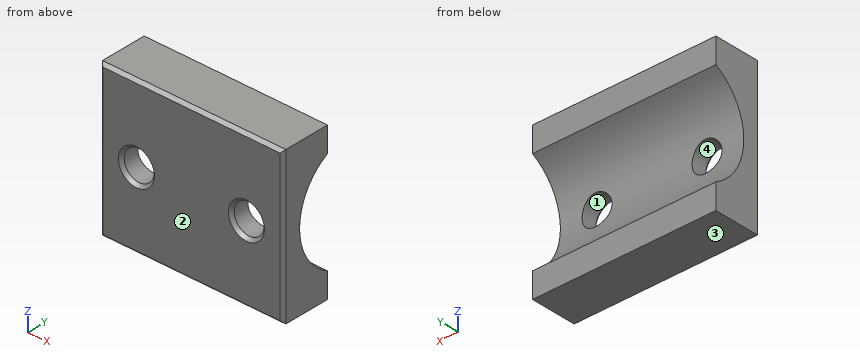
from build123d import *

# Parameters (mm, degrees)
BOSS_EXTRUDE1_DEPTH     = 15
CUT_EXTRUDE1_DEPTH      = 22.100947846
CUT_EXTRUDE1_DEPTH_BACK = 22.100947846
SKETCH2_R               = 2.45
CHAMFER1_SIZE           = 0.5


with BuildPart() as part:
    # Sketch1 → Boss-Extrude1 (new, symmetric)
    with BuildSketch(Plane(origin=(0, 0, 0), x_dir=(0, 0, -1), z_dir=(1, 0, 0))):
        with BuildLine():
            Line((-8.394976176, -4.5), (-12.5, -4.5))
            Line((-12.5, -4.5), (-12.5, -12.5))
            Line((-12.5, -12.5), (12.5, -12.5))
            Line((12.5, -12.5), (12.5, -4.5))
            Line((12.5, -4.5), (8.394976176, -4.5))
            ThreePointArc((8.394976176, -4.5), (0, -9.525), (-8.394976176, -4.5))
        make_face()
    extrude(amount=BOSS_EXTRUDE1_DEPTH, both=True)

    # Sketch2 → Cut-Extrude1 (cut, two sides: drawn at the far end of the back side and taken through both)
    with BuildSketch(Plane.XZ.offset(12.5).offset(-CUT_EXTRUDE1_DEPTH_BACK)):
        with Locations(Location((9, 0, 0), (0, 0, 270))):
            Circle(SKETCH2_R)
        with Locations(Location((-9, 0, 0), (0, 0, 270))):
            Circle(SKETCH2_R)
    extrude(amount=CUT_EXTRUDE1_DEPTH + CUT_EXTRUDE1_DEPTH_BACK, mode=Mode.SUBTRACT)

    # Chamfer1
    chamfer1_edges = [part.edges().sort_by_distance(p)[0] for p in [
        (0, -12.5, -12.5),
        (0, -12.5, 12.5),
        (15, -12.5, 0),
        (-9, -12.5, 2.45),
        (9, -12.5, 2.45),
        (-15, -12.5, 0),
    ]]
    chamfer(chamfer1_edges, length=CHAMFER1_SIZE)


solid = part.part
Part model, mm, in its own coordinate system. Face numbers are marked on the shaded views. Round coordinates to 2 decimals unless told otherwise and drop trailing zeros. Write each loop counter-clockwise with the first axis right and the second up, starting at its lowest first coordinate (ties: lowest second). Pieces come first, ordered by that corner, then holes. Notation, with made-up numbers: M -29,-16.5 L 24,-16.5 A31 ccw 24,11.5 Z; hole C 6.5,40.5 d2. An arc over 180 degrees is marked long. Return JSON: item names as keys, results as strings. Group by question number.
(1) Saw through at D-D on x = 13.5. Write the cut outline in (y, z) (3 decimals), then the cut area to 3 significant figures.
(2) Pin check, flat tips, straight feed: pin 1 Ø8 at (x, z) = (-9, 0) entering from -Y; pin 2 Ø8 at (x, z) = (-8.5, 1.5) entering from +Y; pin 3 Ø4 at (x, z) = (-11.5, -3) entering from +Y. Stop position of each tip, or through.
(3) Saw through at B-B on z = 0. Write the cut outline in (x, y) (3 decimals), then the cut area to 3 significant figures.
(4) Saw through at A-A on x = 9. Write the cut outline in (y, z) (3 decimals).
(5) Drill centre lines: probe 1 along X at (y, z) = (-10.75, 0); probe 2 along Z at (x, y) = (9, -11.05); probe 3 along Z at (x, y) = (-8.5, -4.75). Where is each one in solid material? Low to high.
(6) Two-plate mould, pull along Z, no slides. Class the marked faces 1, 2, 3 and 4: +Z half, -Z half, draft (parallel to the pull), parting line (faces both ways), or undercut.
(7) Saw through at C-C on y = -8.25. Write the cut outline in (x, z), then the cut area to 3 significant figures.
Returned:
{
 "1": {"outline": "M -12.5,-12 L -12,-12.5 L -4.5,-12.5 L -4.5,-8.395 A9.525 cw -4.5,8.395 L -4.5,12.5 L -12,12.5 L -12.5,12 Z", "area": "140 mm²"},
 "2": {"pin 1": "y = -12.5", "pin 2": "y = -7.78", "pin 3": "y = -8.11"},
 "3": {"outline": "M -15,-12 L -14.5,-12.5 L -11.95,-12.5 L -11.45,-12 L -11.45,-9.525 L -15,-9.525 Z; M -6.55,-12 L -6.05,-12.5 L 6.05,-12.5 L 6.55,-12 L 6.55,-9.525 L -6.55,-9.525 Z; M 11.45,-12 L 11.95,-12.5 L 14.5,-12.5 L 15,-12 L 15,-9.525 L 11.45,-9.525 Z", "area": "59.3 mm²"},
 "4": {"outline": "M -12.5,-12 L -12,-12.5 L -4.5,-12.5 L -4.5,-8.395 A9.525 cw -9.205,-2.45 L -12,-2.45 L -12.5,-2.95 Z; M -12.5,2.95 L -12,2.45 L -9.205,2.45 A9.525 cw -4.5,8.395 L -4.5,12.5 L -12,12.5 L -12.5,12 Z"},
 "5": {"probe 1": "-15 to -11.45, -6.55 to 6.55, 11.45 to 15", "probe 2": "-12.5 to -2.45, 2.45 to 12.5", "probe 3": "-12.5 to -8.26, 8.26 to 12.5"},
 "6": {"face 1": "undercut", "face 2": "draft", "face 3": "-Z half", "face 4": "undercut"},
 "7": {"outline": "M -15,-12.5 L 15,-12.5 L 15,-4.76 L -15,-4.76 Z; M -15,4.76 L 15,4.76 L 15,12.5 L -15,12.5 Z", "area": "464 mm²"}
}
